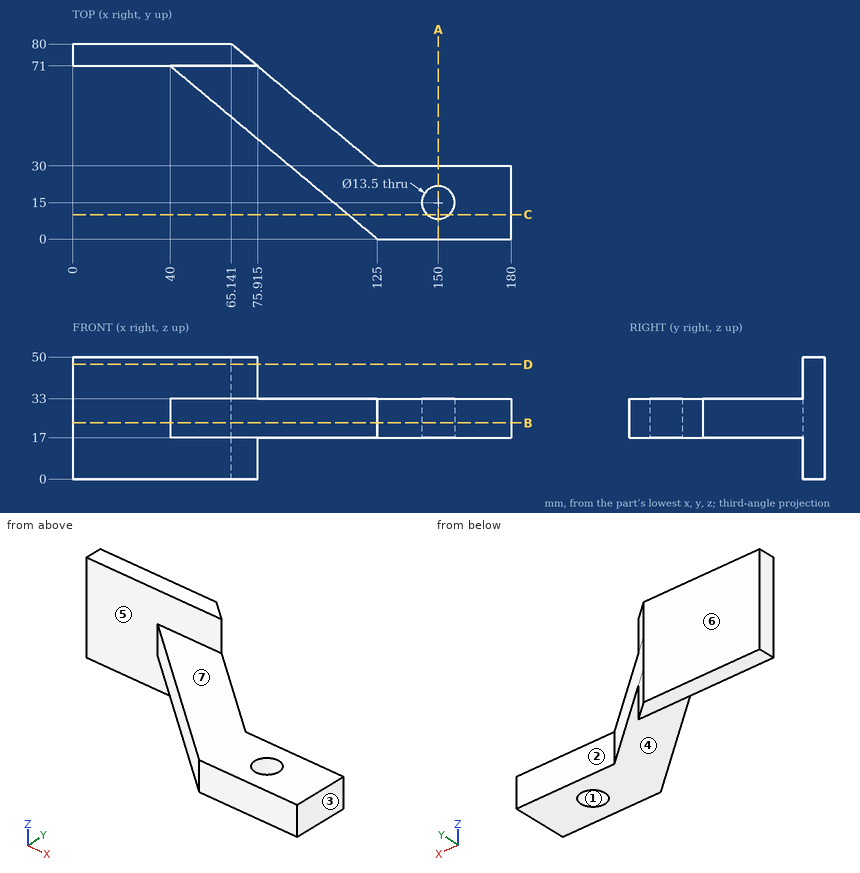
Study the drawing (mm; zero at the part's minimum x, y, z) and answer. A direction names the side the tool comes from. Give positions to 0.01 mm unless a question says otherwise; leave off trailing zeros. Order: outer loops, then holes, each group sorted by start corner. A loop starts at its lowest first (then second) coordinate and runs counter-clockwise, first axis right, second up. Notation, with made-up numbers: (58.25, 83.5) - (66.25, 83.5) arc R32 ccw to (66.25, 121.5) - close; hole circle Ø6 at (20.25, -1.75). An arc over 180 degrees is marked (long way). Answer in a Markdown table with one row per item. Add a question column.
Q1. For a pull along X with two mould halves and no side action, classify the marked faces 1, 2 and 3 as released by +X, released by -X, zero draft, split by the parting line, or undercut.
Q2. The part is cut by section C-C (y = 10). Determine the outline of the cut face in (x, z) (1 decimal).
Q3. The part is cut by section B-B (z = 23). Determine the outline of the cut face in (x, y), then the cut area to 3 significant figures.
Q4. The part is cut by section D-D (z = 47). Determine the outline of the cut face in (x, y) (1 decimal), then the cut area to 3 significant figures.
Q5. Find the intervals of material crossed by line 1 along Y through (x, z) = (150, 21); line 2 along Y through (x, z) = (40.5, 16); line 3 along Z through (x, y) = (167.5, 24), in increasing order. Write a range as [from, to].
Q6. The part is cut by section A-A (x = 150). Determine the outline of the cut face in (y, z), then the cut area to 3 significant figures.
Q7. Which of the six approach directions +Z, -Z, +X, -X, +Y, -Y give full straight-line access (tool end or side, diameter ignored) to the marked faces 4, 5, 6 and 7?
Q8. Given P1, Ø21.5, axis at x = 150, y = 15, coming from the -Z side; P2, Ø4, axis at x = 129, z = 17, coming from the +Y side; P3, Ø1.5, axis at y = 50, z = 21.5, coming from the -X side (1 decimal), each flat-ended and moving along its own axis, determine where each tip first touches the part or whether it passes through.
Determined:
| question | item | result |
|---|---|---|
| 1 | face 1 | undercut |
| 1 | face 2 | zero draft |
| 1 | face 3 | released by +X |
| 2 | outline | (113, 17) - (145.5, 17) - (145.5, 33) - (113, 33) - close; (154.5, 17) - (180, 17) - (180, 33) - (154.5, 33) - close |
| 3 | outline | (0, 71) - (40, 71) - (125, 0) - (180, 0) - (180, 30) - (125, 30) - (65.14, 80) - (0, 80) - close; hole circle Ø13.5 at (150, 15) |
| 3 | area | 4,150 mm² |
| 4 | outline | (0, 71) - (75.9, 71) - (65.1, 80) - (0, 80) - close |
| 4 | area | 635 mm² |
| 5 | line 1 | y = [0, 8.25], [21.75, 30] |
| 5 | line 2 | y = [71, 80] |
| 5 | line 3 | z = [17, 33] |
| 6 | outline | (0, 17) - (8.25, 17) - (8.25, 33) - (0, 33) - close; (21.75, 17) - (30, 17) - (30, 33) - (21.75, 33) - close |
| 6 | area | 264 mm² |
| 7 | face 4 | -Z, +X, -X, -Y |
| 7 | face 5 | -X, -Y |
| 7 | face 6 | +Z, -Z, +X, -X, +Y |
| 7 | face 7 | +Z, +X, -X, -Y |
| 8 | P1 | stops at z = 17 |
| 8 | P2 | stops at y = 30 |
| 8 | P3 | stops at x = 64.2 |
